CAD build for the part. Positions are in the model's coordinates, mm. Face numbers are marked on the shaded views. Give positions to 0.01 mm unless a question says otherwise; leave off trailing zeros. Order: outer loops, then holes, each group sorted by start corner. A loop starts at its lowest first (then second) coordinate and runs counter-clockwise, first axis right, second up.
Item 1: Band-saw the part on D-D on z = 29.5. Give the cut face in (x, y).
Item 2: Flat gauge pins, fed straight in: P1, Ø12, axis at x = 189.5, z = 9, coming from the +Y side; P2, Ø1, axis at x = 116, z = 29, coming from the +Y side; P3, Ø2, axis at y = 131, z = -3, coming from the +X side. Where does each tip first touch, or does it go through?
Item 3: Two-plate mould, pull along X, no slides. Class the marked faces 1, 2 and 3: released by +X, released by -X, zero draft, split by the parting line, or undercut.
Item 4: Band-saw the part on B-B on x = 190. Give the cut face in (y, z) (1 decimal), plus the area to 3 significant figures.
Item 5: Wall check: L1, parallel to X at y = 95.5, z = 26.5; L2, parallel to Y at x = 295, z = 9; L3, parallel to Y at x = 236, z = 24.5. Give the ranges that are in metal, low to high.
Item 6: Band-saw the part on C-C on y = 57. Give the cut face in (x, z).
Item 7: Band-saw the part on A-A on z = 12.5. Give the cut face in (x, y), plus the area to 3 significant figures.
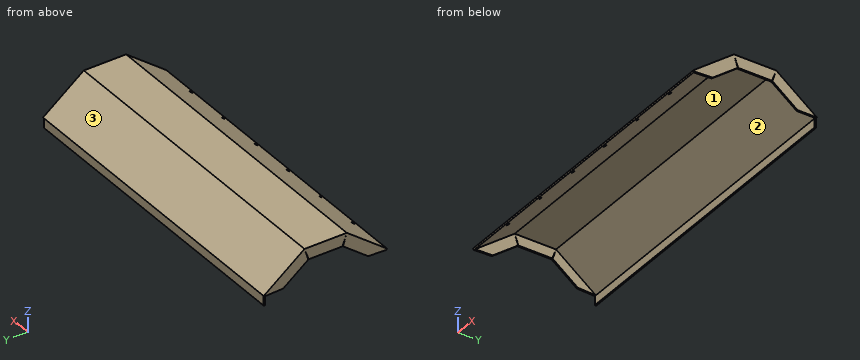
```python
from build123d import *

# Parameters (mm, degrees)
F1_DEPTH  = 342.9
F3_DEPTH  = 1.5875
F4_W      = 1.5875
F4_H      = 10.3091086821
F5_DEPTH  = 25.4
F7_DEPTH  = 1.5875
F9_R      = 1.5875
F10_DEPTH = 1.5875


with BuildPart() as f1:
    # F0 (on Right) → F1 (new body)
    with BuildSketch(Plane.YZ):
        Polygon((-0.9648254583, 1.2606617647), (0, 0), (42.8625, 32.8040655826), (87.3125, 32.8040655826), (130.175, 0), (130.175, -9.525), (131.7625, -9.525), (131.7625, 0.7841086821), (87.8502715669, 34.3915655826), (42.3247284331, 34.3915655826), align=None)
    extrude(amount=F1_DEPTH)

    # F6 (on face) → F7 (join)
    with BuildSketch(Plane(origin=(0, 0, 0), x_dir=(0, -1, 0), z_dir=(-1, 0, 0))):
        Polygon((-130.175, 0), (-110.8146041448, 0.8236222302), (-83.7526464353, 21.5350188005), (-87.3125, 32.8040655826), align=None)
        Polygon((-42.8625, 32.8040655826), (-87.3125, 32.8040655826), (-83.2905208193, 21.6915655826), (-46.8844791807, 21.6915655826), align=None)
        Polygon((0, 0), (-42.8625, 32.8040655826), (-46.4223535647, 21.5350188005), (-19.3603958552, 0.8236222302), align=None)
        Polygon((-130.175, -9.525), (-130.175, 0), (-87.3125, 32.8040655826), (-42.8625, 32.8040655826), (0, 0), (0.9648254583, 1.2606617647), (-42.3247284331, 34.3915655826), (-87.8502715669, 34.3915655826), (-131.7625, 0.7841086821), (-131.7625, -9.525), align=None)
    extrude(amount=F7_DEPTH)


with BuildPart() as f3:
    # F2 (on face) → F3 (new body)
    with BuildSketch(Plane.YZ.offset(342.9)):
        Polygon((0, 0), (19.3603958552, 0.8236222302), (46.4223535647, 21.5350188005), (42.8625, 32.8040655826), align=None)
        Polygon((87.3125, 32.8040655826), (42.8625, 32.8040655826), (46.8844791807, 21.6915655826), (83.2905208193, 21.6915655826), align=None)
        Polygon((130.175, 0), (87.3125, 32.8040655826), (83.7526464353, 21.5350188005), (110.8146041448, 0.8236222302), align=None)
        Polygon((-0.9648254583, 1.2606617647), (0, 0), (42.8625, 32.8040655826), (87.3125, 32.8040655826), (130.175, 0), (130.175, -9.525), (131.7625, -9.525), (131.7625, 0.7841086821), (87.8502715669, 34.3915655826), (42.3247284331, 34.3915655826), align=None)
    extrude(amount=F3_DEPTH)

    # F4 (on face) → F5 (cut)
    with BuildSketch(Plane(origin=(0, 131.7625, 0), x_dir=(-1, 0, 0), z_dir=(0, 1, 0))):
        with Locations((-343.69375, -4.3704456589)):
            Rectangle(F4_W, F4_H)
    extrude(amount=-F5_DEPTH, mode=Mode.SUBTRACT)


with BuildPart() as f1_1:
    add(f1.part)

    # F8: union F3
    add(f3.part)

    # F9 (on face) → F10 (cut, through all)
    with BuildSketch(Plane(origin=(0, -0.9648254583, 1.2606617647), x_dir=(1, 0, 0), z_dir=(0, -0.6077640682, 0.7941176471))):
        with Locations((44.4500253916, 6.35)):
            Circle(F9_R)
        with Locations((95.2500253916, 6.35)):
            Circle(F9_R)
        with Locations((146.0500253916, 6.35)):
            Circle(F9_R)
        with Locations((196.8500253916, 6.35)):
            Circle(F9_R)
        with Locations((247.6500253916, 6.35)):
            Circle(F9_R)
        with Locations((298.4500253916, 6.35)):
            Circle(F9_R)
    extrude(amount=-F10_DEPTH, mode=Mode.SUBTRACT)


solid = f1_1.part
```
The answers:
1. outline: (-1.59, 35.93) - (344.49, 35.93) - (344.49, 43.91) - (342.9, 43.91) - (342.9, 38.55) - (0, 38.55) - (0, 43.91) - (-1.59, 43.91) - close; (-1.59, 44.06) - (0, 44.06) - (0, 86.12) - (-1.59, 86.12) - close; (-1.59, 86.27) - (0, 86.27) - (0, 91.63) - (342.9, 91.63) - (342.9, 86.27) - (344.49, 86.27) - (344.49, 94.24) - (-1.59, 94.24) - close; (342.9, 44.06) - (344.49, 44.06) - (344.49, 86.12) - (342.9, 86.12) - close
2. P1: stops at y = 128.87
2. P2: stops at y = 95.55
2. P3: stops at x = 342.9
3. face 1: undercut
3. face 2: undercut
3. face 3: zero draft
4. outline: (-1, 1.3) - (0, 0) - (42.9, 32.8) - (87.3, 32.8) - (130.2, 0) - (130.2, -9.5) - (131.8, -9.5) - (131.8, 0.8) - (87.9, 34.4) - (42.3, 34.4) - close
4. area: 260 mm2
5. L1: x = -1.59 to 0, 342.9 to 344.49
5. L2: y = 9.15 to 11.76, 118.42 to 121.03
5. L3: y = 29.4 to 32.01, 98.16 to 100.77
6. outline: (-1.59, 21.69) - (0, 21.69) - (0, 32.8) - (342.9, 32.8) - (342.9, 21.69) - (344.49, 21.69) - (344.49, 34.39) - (-1.59, 34.39) - close
7. outline: (-1.59, 13.72) - (344.49, 13.72) - (344.49, 34.62) - (342.9, 34.62) - (342.9, 16.33) - (0, 16.33) - (0, 34.62) - (-1.59, 34.62) - close; (-1.59, 95.56) - (0, 95.56) - (0, 113.84) - (342.9, 113.84) - (342.9, 95.56) - (344.49, 95.56) - (344.49, 116.45) - (-1.59, 116.45) - close
7. area: 1,920 mm2
